from build123d import *

# Parameters (mm, degrees)
F0_W     = 14.7
F0_H     = 13
F1_DEPTH = 11.33
F3_DEPTH = 34


with BuildPart() as f1:
    # F0 (on Top) → F1 (new body)
    with BuildSketch(Plane.XY):
        with Locations((-21.202724, 14.082852)):
            Rectangle(F0_W, F0_H)
    extrude(amount=F1_DEPTH)

    # F2 (on face) → F3 (join)
    with BuildSketch(Plane(origin=(0, 20.582852, 0), x_dir=(-1, 0, 0), z_dir=(0, 1, 0))):
        with BuildLine():
            Line((24.885875, 10.94), (17.519573, 10.94))
            ThreePointArc((17.519573, 10.94), (15.431043, 4.146858), (21.202724, 0))
            ThreePointArc((21.202724, 0), (26.974405, 4.146858), (24.885875, 10.94))
        make_face()
    extrude(amount=-F3_DEPTH)


solid = f1.part
Work out the finished part from the listing and answer in its coordinate system (mm). A direction names the side the tool comes from. Give positions to 0.01 mm unless a question says otherwise; leave off trailing zeros. Order: outer loops, then holes, each group sorted by start corner. A loop starts at its lowest first (then second) coordinate and runs counter-clockwise, first axis right, second up. Notation, with made-up numbers: M -3,-3.5 L 56,-3.5 A31 cw 56,23.5 Z; hole C 46,-15.5 d1. An arc over 180 degrees is marked long. Return JSON: item names as keys, results as strings.
Q1. Find section D-D, the plane x = -14.75. Write down the section's boundary in (y, z).
Answer below:
{"outline": "M 7.58,0 L 20.58,0 L 20.58,11.33 L 7.58,11.33 Z"}
Q2. Find section A-A, the plane x = -19.75. Write down the section's boundary in (y, z), and give its area (3 significant figures).
Answer below:
{"outline": "M -13.42,0.18 L 7.58,0.18 L 7.58,0 L 20.58,0 L 20.58,11.33 L 7.58,11.33 L 7.58,10.94 L -13.42,10.94 Z", "area": "373 mm^2"}
Q3. Each of these flat-tipped pins is pushed along its axis until it touches: pin 1 (3 mm diameter, centred on x = -18.5, y = -8.5, fed in from +Z); pin 2 (2 mm diameter, centred on y = -6.5, z = 8, fed in from -X); pin 3 (2 mm diameter, centred on y = -1, z = 2, fed in from +X). Where does it stop, or does it pass through?
Answer below:
{"pin 1": "stops at z = 10.94", "pin 2": "stops at x = -27.22", "pin 3": "stops at x = -15.95"}
Q4. Find the intervals of material crossed by line 1 along Y through (x, z) = (-14.75, 1.25); line 2 along Z through (x, y) = (-21.25, 2); line 3 along Z through (x, y) = (-23, -4.5), in increasing order. Write a range as [from, to].
Answer below:
{"line 1": "y = [7.58, 20.58]", "line 2": "z = [0, 10.94]", "line 3": "z = [0.27, 10.94]"}
Q5. Find section B-B, the plane z = 0.5. Write down the section's boundary in (x, y).
Answer below:
{"outline": "M -28.55,7.58 L -23.62,7.58 L -23.62,-13.42 L -18.79,-13.42 L -18.79,7.58 L -13.85,7.58 L -13.85,20.58 L -28.55,20.58 Z"}
Q6. Find section C-C, the plane y = -9. Write down the section's boundary in (x, z).
Answer below:
{"outline": "M -24.89,10.94 A6.09 ccw long -17.52,10.94 Z"}
Q7. Which of the six approach directions +Z, -Z, +X, -X, +Y, -Y give full straight-line access (tool end or side, diameter ignored) to faces 1 (the face through (-28.553, 14, 6)), 2 (the face through (-21, -3, 10.94)), 3 (the face through (-25, 7.583, 1))?
Answer below:
{"face 1": "+Z, -Z, -X, +Y, -Y", "face 2": "+Z, +X, -X, -Y", "face 3": "-Y"}
